Input: part model. Units: mm. Frame: model coordinates. A direction names the side the tool comes from. Round coordinates to 2 decimals unless told otherwise and drop trailing zeros. Write each loop counter-clockwise with the first axis right and the second up, starting at its lowest first coordinate (ties: lowest second). Pieces come first, ordered by that corner, then holes. Notation, with made-up numbers: (71.5, 85) - (86.5, 85) arc R17 cw to (86.5, 112) - close; hole circle Ø6 at (62.5, -26.5). An arc over 180 degrees is marked (long way). Use one line per item in the form item = value.
```python
from build123d import *

# Parameters (mm, degrees)
SKETCH1_W           = 812.8
SKETCH1_H           = 101.6
BOSS_EXTRUDE1_DEPTH = 76.2
SKETCH2_W           = 50.8
SKETCH2_H           = 101.6
BOSS_EXTRUDE2_DEPTH = 203.2
SKETCH6_W           = 365.887
SKETCH6_H           = 101.6
BOSS_EXTRUDE5_DEPTH = 50.8
FILLET4_R           = 25.4


with BuildPart() as part:
    # Sketch1 → Boss-Extrude1 (new body)
    with BuildSketch(Plane.XY):
        with Locations((-406.4, 50.8)):
            Rectangle(SKETCH1_W, SKETCH1_H)
    extrude(amount=BOSS_EXTRUDE1_DEPTH)

    # Sketch2 → Boss-Extrude2 (add)
    with BuildSketch(Plane.XY.offset(76.2)):
        with Locations((-838.2, 50.8)):
            Rectangle(SKETCH2_W, SKETCH2_H)
        with Locations((25.4, 50.8)):
            Rectangle(SKETCH2_W, SKETCH2_H)
    extrude(amount=-BOSS_EXTRUDE2_DEPTH)

    # Sketch6 → Boss-Extrude5 (add)
    with BuildSketch(Plane.ZY.offset(863.6)):
        with Locations((-106.7435, 50.8)):
            Rectangle(SKETCH6_W, SKETCH6_H)
    extrude(amount=-BOSS_EXTRUDE5_DEPTH)

    # Fillet4
    fillet4_edges = [part.edges().sort_by_distance(p)[0] for p in [
        (-406.4, 0, 76.2),
        (-812.8, 101.6, -144.8435),
        (-863.6, 101.6, -106.7435),
        (-812.8, 0, -144.8435),
        (-863.6, 0, -106.7435),
        (-863.6, 50.8, 76.2),
        (25.4, 0, -127),
        (50.8, 0, -25.4),
        (0, 0, -63.5),
        (0, 50.8, -127),
        (0, 101.6, -63.5),
        (50.8, 50.8, 76.2),
        (50.8, 101.6, -25.4),
        (25.4, 101.6, -127),
        (50.8, 50.8, -127),
        (-838.2, 101.6, -289.687),
        (-863.6, 50.8, -289.687),
        (-812.8, 50.8, -289.687),
        (-838.2, 0, -289.687),
        (-406.4, 0, 0),
        (-812.8, 50.8, 0),
        (-406.4, 101.6, 0),
        (0, 50.8, 0),
        (-406.4, 101.6, 76.2),
    ]]
    fillet(fillet4_edges, radius=FILLET4_R - 0.0001)  # a hair under: the kernel refuses the full size


solid = part.part
```
(1) Material intervals for L1, parallel to X at y = 51.5, z = -73; L2, parallel to Z at x = -337, y = 26; L3, parallel to X at y = 30, z = -220.5, sorted ascending.
Derived:
L1 = -863.6 to -812.8, 0 to 50.8
L2 = 0 to 76.2
L3 = -863.6 to -812.8
(2) First-contact query: pin 1 Ø6 at (y, z) = (79.5, -93) entering from +X; pin 2 Ø2 at (x, y) = (-500, 11) entering from +Z; pin 3 Ø15 at (y, z) = (54, -122) entering from +X. Flat tips, straight axial feed; report the tip coordinate or a pass-through.
Derived:
pin_1 = 50.8
pin_2 = 72.38
pin_3 = 47.28
(3) Draft query along X for faces 1 (the face through (-820.04, 93.96, -146.52)), 2 (the face through (43.56, 93.96, -26.47)), 3 (the face through (-412.45, 7.64, 68.96)). Return one class per face: released by +X, released by -X, zero draft, split by the parting line, or undercut.
Derived:
face_1 = undercut
face_2 = released by +X
face_3 = zero draft
(4) Cut plane B-B on x = -300. Output: boundary loops of the cut face in (y, z).
Derived:
outline = (0, 25.4) arc R25.4 ccw to (25.4, 0) - (76.2, 0) arc R25.4 ccw to (101.6, 25.4) - (101.6, 50.8) arc R25.4 ccw to (76.2, 76.2) - (25.4, 76.2) arc R25.4 ccw to (0, 50.8) - close
(5) Access query for faces 4 (the face through (7.24, 51.16, -119.36)), 5 (the face through (-401.07, 93.96, 7.24)), 6 (the face through (7.24, 7.64, -64.03)). Directions: +Z, -Z, +X, -X, +Y, -Y. A direction counts if a zero-diameter tool reaches every point of the face in a straight line with its end or side. Return the directions, or none.
Derived:
face_4 = -Z, +Y, -Y
face_5 = -Z, +Y
face_6 = -Z, -Y
